CAD build for the part. Positions are in the model's coordinates, mm. Give positions to 0.01 mm unless a question says otherwise; leave off trailing zeros. Loops run counter-clockwise (first coordinate to the right, second up) from the corner with the lowest first, then second, coordinate; pieces in that order, holes last.
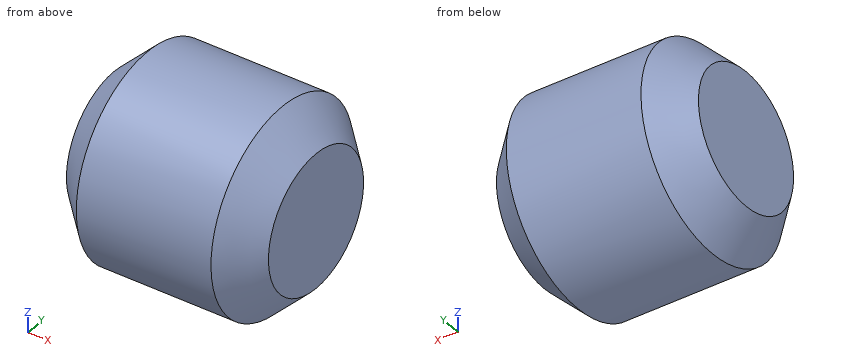
```python
from build123d import *

# Parameters (mm, degrees)
SKETCH1_R           = 300
BOSS_EXTRUDE1_DEPTH = 400
SKETCH1_2_R         = 300
BOSS_EXTRUDE2_DEPTH = 100
BOSS_EXTRUDE2_DRAFT = -45
BOSS_EXTRUDE3_START = 400
SKETCH1_3_R         = 300
BOSS_EXTRUDE3_DEPTH = 100
BOSS_EXTRUDE3_TAPER = 45


with BuildPart() as part:
    # Sketch1 → Boss-Extrude1 (new body)
    with BuildSketch(Plane(origin=(0, 0, 0), x_dir=(0, 0, -1), z_dir=(1, 0, 0))):
        Circle(SKETCH1_R)
    extrude(amount=BOSS_EXTRUDE1_DEPTH)


with BuildPart() as boss_extrude2_tool:
    # Sketch1<2> → Boss-Extrude2 (with draft: the straight prism first)
    with BuildSketch(Plane(origin=(0, 0, 0), x_dir=(0, 0, -1), z_dir=(1, 0, 0))):
        Circle(SKETCH1_2_R)
    extrude(amount=-BOSS_EXTRUDE2_DEPTH)
    # Boss-Extrude2: the draft: its side faces are tilted about the plane it starts from
    boss_extrude2_sides = [boss_extrude2_tool.faces().sort_by_distance(p)[0] for p in [
        (-50, 0, 300),
    ]]
    draft(boss_extrude2_sides, Plane(origin=(0, 0, 0), x_dir=(0, 0, -1), z_dir=(1, 0, 0)), BOSS_EXTRUDE2_DRAFT)


with BuildPart() as part_1:
    add(part.part)

    # Boss-Extrude2: add boss_extrude2_tool
    add(boss_extrude2_tool.part)

    # Sketch1<3> → Boss-Extrude3 (add)
    with BuildSketch(Plane(origin=(0, 0, 0), x_dir=(0, 0, -1), z_dir=(1, 0, 0)).offset(BOSS_EXTRUDE3_START)):
        Circle(SKETCH1_3_R)
    extrude(amount=BOSS_EXTRUDE3_DEPTH, taper=BOSS_EXTRUDE3_TAPER)


solid = part_1.part
```
1. Drop flat-ended pins along their axis: pin 1 (2 mm diameter, centred on y = 223.5, z = -14.5, fed in from +X); pin 2 (12 mm diameter, centred on x = 144, z = -211, fed in from -Y); pin 3 (3 mm diameter, centred on x = 29, z = 187.5, fed in from +Y). Give the stop position or say it passes through.
Responses:
pin 1: stops at x = 477.03
pin 2: stops at y = -219.03
pin 3: stops at y = 235.38
2. Saw through at B-B, the plane x = 313.5. List the corners of the cut face in (y, z), and give its area (3 significant figures).
Responses:
outline: circle Ø600 at (0, 0)
area: 283,000 mm2
3. Saw through at A-A, the plane z = 0. List the corners of the cut face in (x, y), and give its area (3 significant figures).
Responses:
outline: (-100, -200) - (0, -300) - (400, -300) - (500, -200) - (500, 200) - (400, 300) - (0, 300) - (-100, 200) - close
area: 340,000 mm2
4. Saw through at C-C, the plane x = -48.5. List the corners of the cut face in (y, z).
Responses:
outline: circle Ø503 at (0, 0)
5. Probe line 1 along Z through (x, y) = (105, -54.5); line 2 along Z through (x, y) = (179, 187); line 3 along X through (y, z) = (38, 206). List the from-to ranges inside material, lowest first.
Responses:
line 1: z = -295.01 to 295.01
line 2: z = -234.59 to 234.59
line 3: x = -90.52 to 490.52
